CAD build for the part. Positions are in the model's coordinates, mm. A direction names the side the tool comes from. Give positions to 0.01 mm unless a question says otherwise; leave off trailing zeros. Write each loop counter-clockwise with the first axis right and the second up, starting at its lowest first coordinate (ties: lowest second). Pieces come first, ordered by that corner, then holes. Notation, with made-up numbers: (-13, -4.5) - (26, -4.5) arc R34 cw to (26, 29.5) - close; hole circle Ø1 at (-10, 79). An arc over 180 degrees is marked (long way). Answer as a JSON object with one key per item and string values.
from build123d import *

# Parameters (mm, degrees)
F0_W     = 14.224
F0_H     = 69.85
F0_R     = 2.032
F1_DEPTH = 4.953
F0_R_2   = 3.429
F0_R_3   = 1.905
F2_DEPTH = 12.7
F3_DEPTH = 9.906
F0_R_4   = 3.175
F4_DEPTH = 7.747
F5_DEPTH = 19.05
F6_R     = 5.5245
F6_R_2   = 3.429
F7_DEPTH = 6.223


with BuildPart() as f1:
    # F0 (on Top) → F1 (new body)
    with BuildSketch(Plane.XY):
        with Locations((86.868, 34.925)):
            Rectangle(F0_W, F0_H)
        with Locations((90.678, 58.674)):
            Circle(F0_R, mode=Mode.SUBTRACT)
    extrude(amount=F1_DEPTH)

    # F0 (on Top) → F2 (join)
    with BuildSketch(Plane.XY):
        with BuildLine():
            Line((0, 48.514), (0, 0))
            Line((0, 0), (79.756, 0))
            Line((79.756, 0), (79.756, 69.85))
            Line((79.756, 69.85), (12.7, 69.85))
            Line((12.7, 69.85), (12.7, 61.087))
            Line((12.7, 61.087), (40.5765, 61.087))
            ThreePointArc((40.5765, 61.087), (45.021727, 59.245727), (46.863, 54.8005))
            ThreePointArc((46.863, 54.8005), (45.021727, 50.355273), (40.5765, 48.514))
            Line((40.5765, 48.514), (30.902261, 48.514))
            ThreePointArc((30.902261, 48.514), (27.559, 47.117), (24.215739, 48.514))
            Line((24.215739, 48.514), (0, 48.514))
        make_face()
        with Locations((47.879, 26.289)):
            Circle(F0_R_2, mode=Mode.SUBTRACT)
        with Locations((55.626, 45.847)):
            Circle(F0_R_3, mode=Mode.SUBTRACT)
        with Locations((76.962, 53.975)):
            Circle(F0_R_3, mode=Mode.SUBTRACT)
    extrude(amount=F2_DEPTH)

    # F0 (on Top) → F3 (join)
    with BuildSketch(Plane.XY):
        with BuildLine():
            ThreePointArc((12.7, 61.087), (8.935468, 52.188917), (0, 48.514))
            Line((0, 48.514), (24.215739, 48.514))
            ThreePointArc((24.215739, 48.514), (25.774257, 56.162872), (32.258, 51.816))
            ThreePointArc((32.258, 51.816), (31.905872, 50.031257), (30.902261, 48.514))
            Line((30.902261, 48.514), (40.5765, 48.514))
            ThreePointArc((40.5765, 48.514), (45.021727, 50.355273), (46.863, 54.8005))
            ThreePointArc((46.863, 54.8005), (45.021727, 59.245727), (40.5765, 61.087))
            Line((40.5765, 61.087), (12.7, 61.087))
        make_face()
    extrude(amount=F3_DEPTH)

    # F0 (on Top) → F4 (join)
    with BuildSketch(Plane.XY):
        with BuildLine():
            Line((0, 69.85), (0, 48.514))
            ThreePointArc((0, 48.514), (8.935468, 52.188917), (12.7, 61.087))
            Line((12.7, 61.087), (12.7, 69.85))
            Line((12.7, 69.85), (0, 69.85))
        make_face()
        with Locations((6.985, 63.5)):
            Circle(F0_R_4, mode=Mode.SUBTRACT)
    extrude(amount=F4_DEPTH)

    # F0 (on Top) → F5 (join)
    with BuildSketch(Plane.XY):
        with Locations((90.678, 58.674)):
            Circle(F0_R)
    extrude(amount=F5_DEPTH)

    # F6 (on face) → F7 (cut)
    with BuildSketch(Plane.XY):
        with Locations((47.879, 26.289)):
            Circle(F6_R)
        with Locations((47.879, 26.289)):
            Circle(F6_R_2, mode=Mode.SUBTRACT)
    extrude(amount=F7_DEPTH, mode=Mode.SUBTRACT)


solid = f1.part
(1) Saw through at A-A, the plane y = 63.5. Give the cut face in (x, z).
Answer key:
{"outline": "(0, 0) - (3.81, 0) - (3.81, 7.75) - (0, 7.75) - close; (10.16, 0) - (93.98, 0) - (93.98, 4.95) - (79.76, 4.95) - (79.76, 12.7) - (12.7, 12.7) - (12.7, 7.75) - (10.16, 7.75) - close"}
(2) 3-axis set-ups, long thin cutter, end or side, ignore diameter. For faces 1 (the face through (42.36, 26.53, 3.07)), 2 (the face through (12.7, 66, 10)), 3 (the face through (88.648, 58.763, 11.903)), 4 (the face through (26, 61.087, 11)): which of +Z, -Z, +X, -X, +Y, -Y reach the whole face in a straight line?
Answer key:
{"face 1": "-Z", "face 2": "+Z, -X, +Y", "face 3": "+Z", "face 4": "+Z, -X"}
(3) Flat gauge pins, fed straight in: P1, Ø10, axis at x = 28.5, y = 54, coming from the +Z side; P2, Ø4, axis at x = 10.5, y = 45, coming from the +Z side; P3, Ø6.5, axis at x = 7.5, y = 62, coming from the +Z side. Where does each tip first touch, or does it go through?
Answer key:
{"P1": "stops at z = 9.91", "P2": "stops at z = 12.7", "P3": "stops at z = 7.75"}
(4) Saw through at B-B, the plane z = 2.25. State how many separate pieces and enclosed holes the cut face has, and give its area (3 significant figures).
Answer key:
{"separate pieces": "1", "enclosed holes": "5", "area": "6,340 mm²"}
(5) Probe L1, parallel to Y at x = 28, z = 3; L2, parallel to Z at x = 41, y = 21; L3, parallel to X at y = 13, z = 11. List the from-to ranges inside material, lowest first. Write a range as [from, to].
Answer key:
{"L1": "y = [0, 47.14], [56.49, 69.85]", "L2": "z = [0, 12.7]", "L3": "x = [0, 79.76]"}
(6) Pull direction Y, two halves, no side cores. Call faces 5 (the face through (78.722, 53.245, 6.261)), 6 (the face through (46, 0, 6)), 7 (the face through (79.756, 34, 9)), 8 (the face through (54.114, 44.688, 6.261)): pulls with the +Y half, pulls with the -Y half, needs draft (parallel to the pull), parting line crosses it, or undercut.
Answer key:
{"face 5": "undercut", "face 6": "pulls with the -Y half", "face 7": "needs draft", "face 8": "undercut"}
(7) Saw through at C-C, the plane x = 15. Give the cut face in (y, z).
Answer key:
{"outline": "(0, 0) - (69.85, 0) - (69.85, 12.7) - (61.09, 12.7) - (61.09, 9.91) - (48.51, 9.91) - (48.51, 12.7) - (0, 12.7) - close"}
(8) Saw through at D-D, the plane y = 8.5. Give the cut face in (x, z), and give its area (3 significant figures).
Answer key:
{"outline": "(0, 0) - (93.98, 0) - (93.98, 4.95) - (79.76, 4.95) - (79.76, 12.7) - (0, 12.7) - close", "area": "1,080 mm²"}
